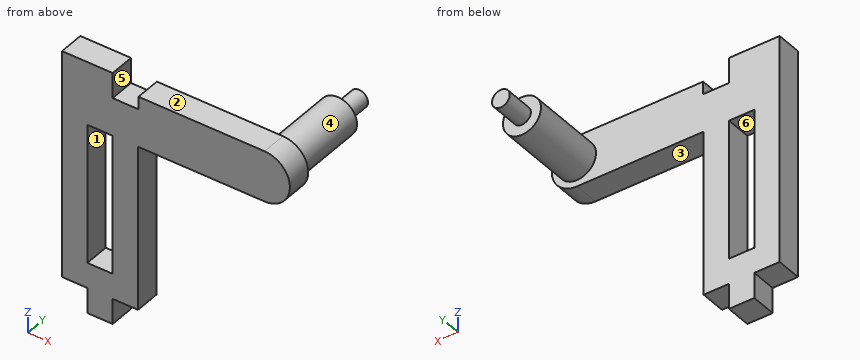
from build123d import *

# Parameters (mm, degrees)
SKETCH2_W           = 5
SKETCH2_H           = 27.5
BOSS_EXTRUDE1_DEPTH = 5
SKETCH3_R           = 3.75
BOSS_EXTRUDE2_DEPTH = 15
SKETCH4_R           = 1.75
BOSS_EXTRUDE3_DEPTH = 5.75


with BuildPart() as part:
    # Sketch2 → Boss-Extrude1 (new body)
    with BuildSketch(Plane(origin=(0, 0, 0), x_dir=(1, 0, 0), z_dir=(0, 1, 0))):
        with BuildLine():
            Line((0, 40), (0, -5))
            Line((0, -5), (10, -5))
            Line((10, -5), (10, 0))
            Line((10, 0), (15.1, 0))
            Line((15.1, 0), (15.1, -2.5))
            Line((15.1, -2.5), (40, -2.5))
            ThreePointArc((40, -2.5), (45, 2.5), (40, 7.5))
            Line((40, 7.5), (15, 7.5))
            Line((15, 7.5), (15, 21.207579156))
            Line((15, 21.207579156), (15, 40))
            Line((15, 40), (10, 40))
            Line((10, 40), (10, 45))
            Line((10, 45), (5, 45))
            Line((5, 45), (5, 40))
            Line((5, 40), (0, 40))
        make_face()
        with Locations((7.5, 21.25)):
            Rectangle(SKETCH2_W, SKETCH2_H, mode=Mode.SUBTRACT)
    extrude(amount=BOSS_EXTRUDE1_DEPTH)

    # Sketch3 → Boss-Extrude2 (add)
    with BuildSketch(Plane(origin=(0, 5, 0), x_dir=(1, 0, 0), z_dir=(0, 1, 0))):
        with Locations(Location((40, 2.5, 0), (0, 0, 270))):
            Circle(SKETCH3_R)
    extrude(amount=BOSS_EXTRUDE2_DEPTH)

    # Sketch4 → Boss-Extrude3 (add)
    with BuildSketch(Plane(origin=(0, 20, 0), x_dir=(1, 0, 0), z_dir=(0, 1, 0))):
        with Locations(Location((40, 2.5, 0), (0, 0, 270))):
            Circle(SKETCH4_R)
    extrude(amount=BOSS_EXTRUDE3_DEPTH)


solid = part.part
Build history of the part. All positions in model axes, mm. Face numbers are marked on the shaded views. A direction names the side the tool comes from. Coordinates: 2 decimals unless noted, no trailing zeros. Write each loop counter-clockwise with the first axis right and the second up, starting at its lowest first coordinate (ties: lowest second). Pieces come first, ordered by that corner, then holes. Notation, with made-up numbers: (51.25, -8.5) -> (80.25, -8.5) arc R16 ccw to (80.25, 20.5) -> close; hole circle Ø1 at (15.25, 50). An arc over 180 degrees is marked (long way). Use CSV: the item, a comma, the result in double quotes. Start each with the question number.
Q1. Pull direction Z, two halves, no side cores. Call the marked faces 4, 5 and 6: released by +Z, released by -Z, zero draft, split by the parting line, or undercut.
Q2. Cut at A-A, the plane z = -17. List the corners of the cut face in (x, y).
Q3. Cut at B-B, the plane y = 2.75. List the corners of the cut face in (x, z), then the cut area to 3 significant figures.
Q4. Cut at C-C, the plane z = -2.5. List the corners of the cut face in (x, y), then the cut area to 3 significant figures.
Q5. Drill centre lines: probe 1 along X at (y, z) = (1.25, -16); probe 2 along Z at (x, y) = (6, 2); probe 3 along Y at (x, z) = (32, -1.5). Where is each one in solid material? Low to high.
Q6. Flat gauge pins, fed straight in: pin 1 Ø5.5 at (y, z) = (2.5, -24.5) entering from +X; pin 2 Ø1.5 at (y, z) = (3, -41.5) entering from +X; pin 3 Ø4 at (x, y) = (13, 3.5) entering from -Z. Where does each tip first touch, or does it go through?
Q7. Cut at D-D, the plane x = 39. List the corners of the cut face in (y, z).
Q8. 3-axis set-ups, long thin cutter, end or side, ignore diameter. For the marked faces 1, 2 and 3: which of +Z, -Z, +X, -X, +Y, -Y reach the whole face in a straight line?
Checked values:
1,face 4,"split by the parting line"
1,face 5,"zero draft"
1,face 6,"undercut"
2,outline,"(0, 0) -> (5, 0) -> (5, 5) -> (0, 5) -> close; (10, 0) -> (15, 0) -> (15, 5) -> (10, 5) -> close"
3,outline,"(0, -40) -> (5, -40) -> (5, -45) -> (10, -45) -> (10, -40) -> (15, -40) -> (15, -7.5) -> (40, -7.5) arc R5 ccw to (40, 2.5) -> (15.1, 2.5) -> (15.1, 0) -> (10, 0) -> (10, 5) -> (0, 5) -> close; hole (5, -35) -> (10, -35) -> (10, -7.5) -> (5, -7.5) -> close"
3,area,"827 mm²"
4,outline,"(0, 0) -> (45, 0) -> (45, 5) -> (43.75, 5) -> (43.75, 20) -> (41.75, 20) -> (41.75, 25.75) -> (38.25, 25.75) -> (38.25, 20) -> (36.25, 20) -> (36.25, 5) -> (0, 5) -> close"
4,area,"358 mm²"
5,probe 1,"x = 0 to 5, 10 to 15"
5,probe 2,"z = -45 to -35, -7.5 to 5"
5,probe 3,"y = 0 to 5"
6,pin 1,"stops at x = 15"
6,pin 2,"stops at x = 10"
6,pin 3,"stops at z = -40"
7,outline,"(0, -7.5) -> (5, -7.5) -> (5, -6.11) -> (20, -6.11) -> (20, -3.94) -> (25.75, -3.94) -> (25.75, -1.06) -> (20, -1.06) -> (20, 1.11) -> (5, 1.11) -> (5, 2.5) -> (0, 2.5) -> close"
8,face 1,"+Y, -Y"
8,face 2,"+Z, +X, +Y, -Y"
8,face 3,"-Z, +X, +Y, -Y"
